from build123d import *

# Parameters (mm, degrees)
SKETCH_W     = 15
SKETCH_H     = 10
PAD_DEPTH    = 3
SKETCH001_W  = 3
SKETCH001_H  = 10
PAD001_DEPTH = 22
SKETCH002_R  = 1.05
POCKET_DEPTH = 6.001
FILLET_R     = 3
FILLET001_R  = 3
FILLET002_R  = 1
FILLET003_R  = 1


with BuildPart() as part:
    # Sketch → Pad (new body)
    with BuildSketch(Plane.XY):
        with Locations((-2.5, -2)):
            Rectangle(SKETCH_W, SKETCH_H)
        with BuildLine():
            ThreePointArc((1.55, 0), (0, 1.55), (-1.55, 0))
            Line((-1.55, 0), (-1.55, -3))
            ThreePointArc((-1.55, -3), (0, -4.55), (1.55, -3))
            Line((1.55, 0), (1.55, -3))
        make_face(mode=Mode.SUBTRACT)
    extrude(amount=PAD_DEPTH)

    # Sketch001 → Pad001 (new body)
    with BuildSketch(Plane.XY.offset(3)):
        with Locations((-5.5, -2)):
            Rectangle(SKETCH001_W, SKETCH001_H)
    extrude(amount=PAD001_DEPTH)

    # Sketch002 → Pocket (cut, through all)
    with BuildSketch(Plane.YZ.offset(-4)):
        with Locations((-4, 19.8)):
            Circle(SKETCH002_R)
        with Locations((-4, 10)):
            Circle(SKETCH002_R)
    extrude(amount=-POCKET_DEPTH, mode=Mode.SUBTRACT)

    # Fillet
    fillet_edges = [part.edges().sort_by_distance(p)[0] for p in [
        (-10, -7, 1.5),
        (-10, 3, 1.5),
        (5, -7, 1.5),
        (5, 3, 1.5),
    ]]
    fillet(fillet_edges, radius=FILLET_R)

    # Fillet001
    fillet001_edges = [part.edges().sort_by_distance(p)[0] for p in [
        (-5.5, -7, 25),
        (-5.5, 3, 25),
    ]]
    fillet(fillet001_edges, radius=FILLET001_R)

    # Fillet002
    fillet002_edges = [part.edges().sort_by_distance(p)[0] for p in [
        (-4, -2, 3),
    ]]
    fillet(fillet002_edges, radius=FILLET002_R)

    # Fillet003
    fillet003_edges = [part.edges().sort_by_distance(p)[0] for p in [
        (-4, -6.12132, 24.12132),
    ]]
    fillet(fillet003_edges, radius=FILLET003_R)


solid = part.part
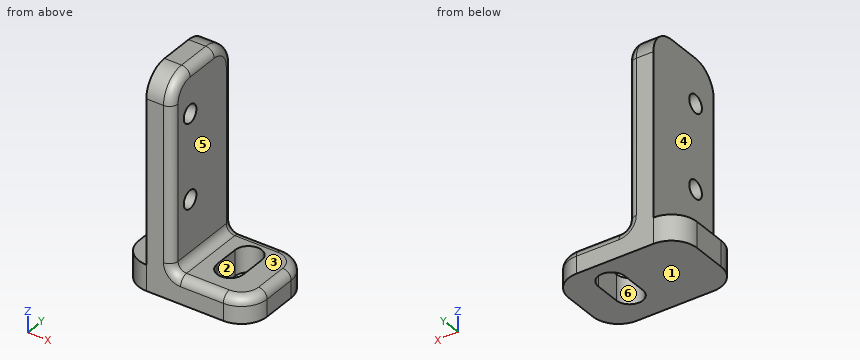
Here's how the part is built. I have some questions about the finished solid (model axes, mm). Face numbers are marked on the shaded views. A direction names the side the tool comes from. Round coordinates to 2 decimals unless told otherwise and drop trailing zeros. Write each loop counter-clockwise with the first axis right and the second up, starting at its lowest first coordinate (ties: lowest second). Pieces come first, ordered by that corner, then holes. Notation, with made-up numbers: (-18, 84.25) -> (-11, 84.25) arc R23 cw to (-11, 103.25) -> close; hole circle Ø9 at (8.5, 41.25). An arc over 180 degrees is marked (long way). One line per item, written item: value.
1) Suppose I cut it at C-C on z = 10. List the corners of the cut face in (x, y) for me.
Filled sheet:
outline: (-7, -7) -> (-5, -7) arc R1 ccw to (-4, -6) -> (-4, -5.05) -> (-7, -5.05) -> close; (-7, -2.95) -> (-4, -2.95) -> (-4, 2) arc R1 ccw to (-5, 3) -> (-7, 3) -> close
2) I'm going to push flat-ended pins straight in: pin 1 Ø4 at (y, z) = (-0.5, 14.5) entering from +X; pin 2 Ø5 at (y, z) = (-1, 8.5) entering from -X; pin 3 Ø5.5 at (x, y) = (0, -3.5) entering from +Z. Where does each tip first touch, or does it pass through?
Filled sheet:
pin 1: stops at x = -4
pin 2: stops at x = -7
pin 3: stops at z = 3
3) If I drill on line 1 (Z direction, x = -5.6, y = -4); line 2 (X direction, y = 0, z = 21.25); line 3 (Z direction, x = -8.5, y = -5.5), over which ranges is the centre line in solid material (lowest first)? Write a range as [from, to].
Filled sheet:
line 1: z = [0, 8.95], [11.05, 18.75], [20.85, 25]
line 2: x = [-7, -4]
line 3: z = [0, 3]
4) Suppose I cut it at D-D on x = -5.5. List the corners of the cut face in (y, z) for me, plus the area to 3 significant figures.
Filled sheet:
outline: (-7, 0) -> (3, 0) -> (3, 22) arc R3 ccw to (0, 25) -> (-4, 25) arc R3 ccw to (-7, 22) -> close; hole circle Ø2.1 at (-4, 10); hole circle Ø2.1 at (-4, 19.8)
area: 239 mm2
5) Suppose I cut it at B-B on y = -0.5. List the corners of the cut face in (x, z) for me.
Filled sheet:
outline: (-10, 0) -> (-1.55, 0) -> (-1.55, 3) -> (-3, 3) arc R1 cw to (-4, 4) -> (-4, 24) arc R1 ccw to (-5, 25) -> (-7, 25) -> (-7, 3) -> (-10, 3) -> close; (1.55, 0) -> (5, 0) -> (5, 2) arc R1 ccw to (4, 3) -> (1.55, 3) -> close
6) Suppose I cut it at A-A on x = 0. List the corners of the cut face in (y, z) for me, plus the area to 3 significant figures.
Filled sheet:
outline: (-7, 0) -> (-4.55, 0) -> (-4.55, 3) -> (-6, 3) arc R1 ccw to (-7, 2) -> close; (1.55, 0) -> (3, 0) -> (3, 2) arc R1 ccw to (2, 3) -> (1.55, 3) -> close
area: 11.3 mm2
7) We'd pull the mould along X, two halves only. Please class the marked faces 4, 5 and 6: released by +X, released by -X, zero draft, split by the parting line, or undercut.
Filled sheet:
face 4: released by -X
face 5: released by +X
face 6: undercut
8) For the marked faces 1, 2 and 3, which set-ups out of +Z, -Z, +X, -X, +Y, -Y let a thin tool reach every point of the face, with its end or its side?
Filled sheet:
face 1: -Z, +X, -X, +Y, -Y
face 2: +Z, -Z
face 3: +Z, +X, +Y, -Y
